```python
from build123d import *

# Parameters (mm, degrees)
BOSS_EXTRUDE1_DEPTH = 15
SKETCH3_R           = 1.5
CUT_EXTRUDE1_DEPTH  = 3
CUT_EXTRUDE2_REACH  = 29.821
SKETCH4_R           = 2.5
FILLET1_R           = 1


with BuildPart() as part:
    # Sketch1 → Boss-Extrude1 (new, symmetric)
    with BuildSketch(Plane.XY):
        Polygon((-6, 0), (6, 0), (6, 15), (9, 15), (9, -3), (-9, -3), (-9, 15), (-6, 15), align=None)
    extrude(amount=BOSS_EXTRUDE1_DEPTH, both=True)

    # Sketch3 → Cut-Extrude1 (cut)
    with BuildSketch(Plane(origin=(0, 0, 0), x_dir=(1, 0, 0), z_dir=(0, 1, 0))):
        with Locations(Location((0, 10, 0), (0, 0, 270))):
            Circle(SKETCH3_R)
        with Locations(Location((0, -10, 0), (0, 0, 90))):
            Circle(SKETCH3_R)
    extrude(amount=-CUT_EXTRUDE1_DEPTH, mode=Mode.SUBTRACT)

    # Cut-Extrude2: up to this face of the body (flat: up to its plane)
    cut_extrude2_end = Plane(part.part.faces().sort_by_distance((-9, 6, 0))[0])
    # Sketch4 → Cut-Extrude2 (cut, up to the picked face)
    with BuildSketch(Plane(origin=(9, 0, 0), x_dir=(0, 0, -1), z_dir=(1, 0, 0)), mode=Mode.PRIVATE) as cut_extrude2_sk1:
        with Locations(Location((0, 10, 0), (0, 0, 90))):
            Circle(SKETCH4_R)
    cut_extrude2_tool1 = split(extrude(cut_extrude2_sk1.sketch, amount=-CUT_EXTRUDE2_REACH, mode=Mode.PRIVATE), bisect_by=cut_extrude2_end, keep=Keep.BOTH, mode=Mode.PRIVATE)
    # Sketch4 → Cut-Extrude2 (cut, up to the picked face)
    with BuildSketch(Plane(origin=(9, 0, 0), x_dir=(0, 0, -1), z_dir=(1, 0, 0)), mode=Mode.PRIVATE) as cut_extrude2_sk2:
        Polygon((-15, 15), (-5, 15), (-15, 5), align=None)
    cut_extrude2_tool2 = split(extrude(cut_extrude2_sk2.sketch, amount=-CUT_EXTRUDE2_REACH, mode=Mode.PRIVATE), bisect_by=cut_extrude2_end, keep=Keep.BOTH, mode=Mode.PRIVATE)
    # Sketch4 → Cut-Extrude2 (cut, up to the picked face)
    with BuildSketch(Plane(origin=(9, 0, 0), x_dir=(0, 0, -1), z_dir=(1, 0, 0)), mode=Mode.PRIVATE) as cut_extrude2_sk3:
        Polygon((15, 5), (5, 15), (15, 15), align=None)
    cut_extrude2_tool3 = split(extrude(cut_extrude2_sk3.sketch, amount=-CUT_EXTRUDE2_REACH, mode=Mode.PRIVATE), bisect_by=cut_extrude2_end, keep=Keep.BOTH, mode=Mode.PRIVATE)
    add(cut_extrude2_tool1.solids().sort_by(Axis((9, 10, 0), (-1, 0, 0)))[0], mode=Mode.SUBTRACT)
    add(cut_extrude2_tool2.solids().sort_by(Axis((9, 11.666667, 11.666667), (-1, 0, 0)))[0], mode=Mode.SUBTRACT)
    add(cut_extrude2_tool3.solids().sort_by(Axis((9, 11.666667, -11.666667), (-1, 0, 0)))[0], mode=Mode.SUBTRACT)

    # Fillet1
    fillet1_edges = [part.edges().sort_by_distance(p)[0] for p in [
        (-6, 0, 0),
        (6, 0, 0),
    ]]
    fillet(fillet1_edges, radius=FILLET1_R)


solid = part.part
```
Part model, mm, in its own coordinate system. A direction names the side the tool comes from. Round coordinates to 2 decimals unless told otherwise and drop trailing zeros. Write each loop counter-clockwise with the first axis right and the second up, starting at its lowest first coordinate (ties: lowest second). Pieces come first, ordered by that corner, then holes.
Item 1: Cut at A-A, the plane x = 0. Give the cut face in (y, z), plus the area to 3 significant figures.
Results:
outline: (-3, -15) - (0, -15) - (0, -11.5) - (-3, -11.5) - close; (-3, -8.5) - (0, -8.5) - (0, 8.5) - (-3, 8.5) - close; (-3, 11.5) - (0, 11.5) - (0, 15) - (-3, 15) - close
area: 72.0 mm2
Item 2: Cut at B-B, the plane y = 3. Give the cut face in (x, z), plus the area to 3 significant figures.
Results:
outline: (-9, -15) - (-6, -15) - (-6, 15) - (-9, 15) - close; (6, -15) - (9, -15) - (9, 15) - (6, 15) - close
area: 180 mm2
Item 3: Probe L1, parallel to X at y = 12.75, z = 6; L2, parallel to Z at x = -6.6, y = 10; L3, parallel to Y at x = 0.25, z = 4. List the from-to ranges inside material, lowest first.
Results:
L1: x = -9 to -6, 6 to 9
L2: z = -10 to -2.5, 2.5 to 10
L3: y = -3 to 0
Item 4: Drop flat-ended pins along their axis: pin 1 Ø5 at (x, z) = (0, -10) entering from -Y; pin 2 Ø8 at (x, y) = (6, 13) entering from -Z; pin 3 Ø2 at (x, z) = (-1.5, 0.5) entering from +Y; pin 4 Ø1.5 at (x, y) = (-5, 7) entering from -Z. Give the stop position or say it passes through.
Results:
pin 1: stops at y = -3
pin 2: stops at z = -11
pin 3: stops at y = 0
pin 4: passes through
Item 5: Cut at D-D, the plane y = 10. Give the cut face in (x, z).
Results:
outline: (-9, -10) - (-6, -10) - (-6, -2.5) - (-9, -2.5) - close; (-9, 2.5) - (-6, 2.5) - (-6, 10) - (-9, 10) - close; (6, -10) - (9, -10) - (9, -2.5) - (6, -2.5) - close; (6, 2.5) - (9, 2.5) - (9, 10) - (6, 10) - close
Item 6: Two-plate mould, pull along X, no slides. Class faces 1 (the flat face through (6, 6, 0)), 2 (the flat face through (-9, 4, 0)), 3 (the flat face through (-7, 10, 10)): +X half, -X half, draft (parallel to the pull), parting line (faces both ways), or undercut.
Results:
face 1: undercut
face 2: -X half
face 3: draft
Item 7: Cut at C-C, the plane z = 10. Give the cut face in (x, y), plus the area to 3 significant figures.
Results:
outline: (-9, -3) - (-1.5, -3) - (-1.5, 0) - (-5, 0) arc R1 cw to (-6, 1) - (-6, 10) - (-9, 10) - close; (1.5, -3) - (9, -3) - (9, 10) - (6, 10) - (6, 1) arc R1 cw to (5, 0) - (1.5, 0) - close
area: 105 mm2
Item 8: Which spindle directions (+Z, -Z, +X, -X, +Y, -Y) get a long thin tool onto all of the face, cutting with end or side? Do faces 4 (the flat face through (8, 10, 10)), 5 (the cylindrical face through (-5.699, 0.285, 0.21)). Say none if no direction does.
Results:
face 4: +Z, +X, -X, +Y
face 5: +Z, -Z, +Y
